Design review of the part shown in the three views and the two pictorial views. Dimensions are in mm from the part's minimum x, y and z. Coordinates: 2 decimals unless noted, no trailing zeros. Write each loop counter-clockwise with the first axis right and the second up, starting at its lowest first coordinate (ties: lowest second). Pieces come first, ordered by that corner, then holes. Notation, with made-up numbers: (19.5, -27.5) - (38.5, -27.5) arc R21 cw to (38.5, 11.5) - close; hole circle Ø6 at (63, 45.5). An arc over 180 degrees is marked (long way). Answer as CSV lines item,"result". Start each with the question number.
Q1. We need section A-A (y = 22.25). Write out the cut boundary in (x, z) (3 decimals), plus the area to 3 significant figures.
Q2. We need section B-B (z = 190.5). Write out the cut boundary in (x, y) (3 decimals).
Q3. Clearance check with flat-ended pins moving along their axes: pin 1 (1.5 mm diameter, centred on x = 28.5, z = 51, fed in from +Y) (3 decimals); pin 2 (3 mm diameter, centred on x = 4, z = 153, fed in from +Y); pin 3 (2.5 mm diameter, centred on x = 37, y = 14.5, fed in from +Z); pin 4 (5 mm diameter, centred on x = 20.5, y = 6, fed in from +Z). State where each tip first meets the part, or that it passes through.
Q4. For line 1 along Y through (x, z) = (1.5, 116.84); line 2 along X through (y, z) = (21.25, 33) (3 decimals); line 3 along Y through (x, z) = (22, 142) (3 decimals), list the stretches that pass through material, from the lowest coordinate up. Write a range as [from, to].
Q5. We need section C-C (x = 17.5). Write out the cut boundary in (y, z) (3 decimals).
Q6. Mouldability with a two-part tool opening along X and no side actions: class the marked faces 1, 2, 3 and 4 as pulls with the +X half, pulls with the -X half, needs draft (parallel to the pull), parting line crosses it, or undercut.
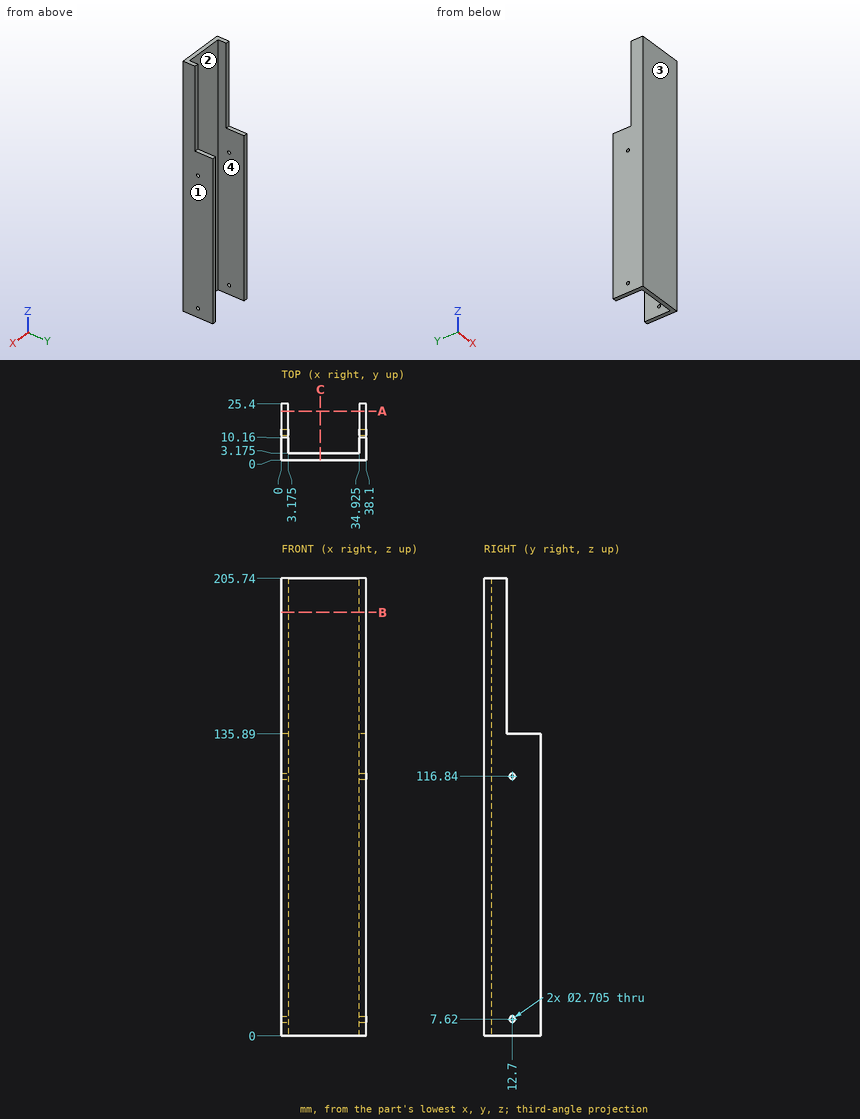
Results list:
1,outline,"(0, 0) - (3.175, 0) - (3.175, 135.89) - (0, 135.89) - close; (34.925, 0) - (38.1, 0) - (38.1, 135.89) - (34.925, 135.89) - close"
1,area,"863 mm2"
2,outline,"(0, 0) - (38.1, 0) - (38.1, 10.16) - (34.925, 10.16) - (34.925, 3.175) - (3.175, 3.175) - (3.175, 10.16) - (0, 10.16) - close"
3,pin 1,"stops at y = 3.175"
3,pin 2,"stops at y = 10.16"
3,pin 3,"stops at z = 135.89"
3,pin 4,"passes through"
4,line 1,"y = [0, 11.35], [14.05, 25.4]"
4,line 2,"x = [0, 3.175], [34.925, 38.1]"
4,line 3,"y = [0, 3.175]"
5,outline,"(0, 0) - (3.175, 0) - (3.175, 205.74) - (0, 205.74) - close"
6,face 1,"pulls with the +X half"
6,face 2,"undercut"
6,face 3,"needs draft"
6,face 4,"undercut"
